Model file for the job. Use its own axes, mm. A direction names the side the tool comes from. Round coordinates to 2 decimals unless told otherwise and drop trailing zeros. Write each loop counter-clockwise with the first axis right and the second up, starting at its lowest first coordinate (ties: lowest second). Pieces come first, ordered by that corner, then holes. Notation, with made-up numbers: (-19, -35) - (23, -35) arc R21 ccw to (23, -20) - close; hole circle Ø9 at (67, -16.75). An arc over 180 degrees is marked (long way). One line per item, written item: value.
from build123d import *

# Parameters (mm, degrees)
F0_R      = 45
F1_DEPTH  = 10
F2_R      = 24.5
F2_R_2    = 20
F3_DEPTH  = 140
F4_R      = 45
F4_R_2    = 24.5
F4_R_3    = 20
F5_DEPTH  = 10
F8_DEPTH  = 195
F10_DEPTH = 18.5
F11_R     = 18.499
F12_R     = 28.5
F13_DEPTH = 10
F15_DEPTH = 25
F16_R     = 14
F17_DEPTH = 99.7
F18_R     = 20
F19_DEPTH = 202.6


# Not quite as in the source:
# - a fillet or chamfer is up to 0.001 mm smaller than in the source, because OpenCascade refuses the exact size


with BuildPart() as f1:
    # F0 (on Top) → F1 (new body)
    with BuildSketch(Plane.XY):
        Circle(F0_R)
    extrude(amount=F1_DEPTH)

    # F2 (on face) → F3 (join)
    with BuildSketch(Plane.XY.offset(10)):
        Circle(F2_R)
        Circle(F2_R_2, mode=Mode.SUBTRACT)
        Circle(F2_R_2)
    extrude(amount=F3_DEPTH)

    # F4 (on face) → F5 (join)
    with BuildSketch(Plane.XY.offset(150)):
        Circle(F4_R)
        Circle(F4_R_2, mode=Mode.SUBTRACT)
        Circle(F4_R_2)
        Circle(F4_R_3, mode=Mode.SUBTRACT)
        Circle(F4_R_3)
    extrude(amount=F5_DEPTH)

    # F7 (on face) → F8 (cut)
    with BuildSketch(Plane(origin=(0, 0, 0), x_dir=(1, 0, 0), z_dir=(0, 0, -1))):
        with BuildLine():
            ThreePointArc((-34.7419642857, -4.2421595409), (-35, 0), (-34.7419642857, 4.2421595409))
            ThreePointArc((-34.7419642857, 4.2421595409), (-39.25, 0), (-34.7419642857, -4.2421595409))
        make_face()
        with BuildLine():
            ThreePointArc((-30.75, 0), (-31.904911004, 2.9125459837), (-34.7419642857, 4.2421595409))
            ThreePointArc((-34.7419642857, 4.2421595409), (-35, 0), (-34.7419642857, -4.2421595409))
            ThreePointArc((-34.7419642857, -4.2421595409), (-31.904911004, -2.9125459837), (-30.75, 0))
        make_face()
        with BuildLine():
            ThreePointArc((-4.2421595409, -34.7419642857), (0, -35), (4.2421595409, -34.7419642857))
            ThreePointArc((4.2421595409, -34.7419642857), (0, -30.75), (-4.2421595409, -34.7419642857))
        make_face()
        with BuildLine():
            ThreePointArc((4.25, -35), (4.248039433, -34.8709225982), (4.2421595409, -34.7419642857))
            ThreePointArc((4.2421595409, -34.7419642857), (0, -35), (-4.2421595409, -34.7419642857))
            ThreePointArc((-4.2421595409, -34.7419642857), (-0.1290774018, -39.248039433), (4.25, -35))
        make_face()
        with BuildLine():
            ThreePointArc((34.7419642857, -4.2421595409), (34.935431513, -2.125), (35, 0))
            ThreePointArc((35, 0), (34.935431513, 2.125), (34.7419642857, 4.2421595409))
            ThreePointArc((34.7419642857, 4.2421595409), (30.75, 0), (34.7419642857, -4.2421595409))
        make_face()
        with BuildLine():
            ThreePointArc((34.7419642857, 4.2421595409), (34.935431513, 2.125), (35, 0))
            ThreePointArc((35, 0), (34.935431513, -2.125), (34.7419642857, -4.2421595409))
            ThreePointArc((34.7419642857, -4.2421595409), (37.9125459837, -3.095088996), (39.25, 0))
            ThreePointArc((39.25, 0), (37.9125459837, 3.095088996), (34.7419642857, 4.2421595409))
        make_face()
        with BuildLine():
            ThreePointArc((24.7487373415, 24.7487373415), (26.2056824365, 23.2004786165), (27.5659383164, 21.5666187599))
            ThreePointArc((27.5659383164, 21.5666187599), (28.6240182438, 23.0038310608), (28.9987373415, 24.7487373415))
            ThreePointArc((28.9987373415, 24.7487373415), (26.2551396829, 28.7228098102), (21.5666187599, 27.5659383164))
            ThreePointArc((21.5666187599, 27.5659383164), (23.2004786165, 26.2056824365), (24.7487373415, 24.7487373415))
        make_face()
        with BuildLine():
            ThreePointArc((21.7435335215, 21.7435335215), (24.6196599397, 20.5006979085), (27.5659383164, 21.5666187599))
            ThreePointArc((27.5659383164, 21.5666187599), (26.2056824365, 23.2004786165), (24.7487373415, 24.7487373415))
            Line((24.7487373415, 24.7487373415), (21.7435335215, 21.7435335215))
        make_face()
        with BuildLine():
            Line((21.7435335215, 21.7435335215), (24.7487373415, 24.7487373415))
            ThreePointArc((24.7487373415, 24.7487373415), (23.2004786165, 26.2056824365), (21.5666187599, 27.5659383164))
            ThreePointArc((21.5666187599, 27.5659383164), (20.5006979085, 24.6196599397), (21.7435335215, 21.7435335215))
        make_face()
        with BuildLine():
            ThreePointArc((28.9987373415, -24.7487373415), (28.6240182438, -23.0038310608), (27.5659383164, -21.5666187599))
            ThreePointArc((27.5659383164, -21.5666187599), (26.2056824365, -23.2004786165), (24.7487373415, -24.7487373415))
            ThreePointArc((24.7487373415, -24.7487373415), (23.2004786165, -26.2056824365), (21.5666187599, -27.5659383164))
            ThreePointArc((21.5666187599, -27.5659383164), (26.2551396829, -28.7228098102), (28.9987373415, -24.7487373415))
        make_face()
        with BuildLine():
            ThreePointArc((21.5666187599, -27.5659383164), (23.2004786165, -26.2056824365), (24.7487373415, -24.7487373415))
            Line((24.7487373415, -24.7487373415), (21.7435335215, -21.7435335215))
            ThreePointArc((21.7435335215, -21.7435335215), (20.5006979085, -24.6196599397), (21.5666187599, -27.5659383164))
        make_face()
        with BuildLine():
            ThreePointArc((24.7487373415, -24.7487373415), (26.2056824365, -23.2004786165), (27.5659383164, -21.5666187599))
            ThreePointArc((27.5659383164, -21.5666187599), (24.6196599397, -20.5006979085), (21.7435335215, -21.7435335215))
            Line((21.7435335215, -21.7435335215), (24.7487373415, -24.7487373415))
        make_face()
        with BuildLine():
            ThreePointArc((-27.5659383164, -21.5666187599), (-27.7539411616, -27.7539411616), (-21.5666187599, -27.5659383164))
            ThreePointArc((-21.5666187599, -27.5659383164), (-23.2004786165, -26.2056824365), (-24.7487373415, -24.7487373415))
            ThreePointArc((-24.7487373415, -24.7487373415), (-26.2056824365, -23.2004786165), (-27.5659383164, -21.5666187599))
        make_face()
        with BuildLine():
            Line((-24.7487373415, -24.7487373415), (-21.7435335215, -21.7435335215))
            ThreePointArc((-21.7435335215, -21.7435335215), (-24.6196599397, -20.5006979085), (-27.5659383164, -21.5666187599))
            ThreePointArc((-27.5659383164, -21.5666187599), (-26.2056824365, -23.2004786165), (-24.7487373415, -24.7487373415))
        make_face()
        with BuildLine():
            ThreePointArc((-20.4987373415, -24.7487373415), (-20.8222493284, -23.122332754), (-21.7435335215, -21.7435335215))
            Line((-21.7435335215, -21.7435335215), (-24.7487373415, -24.7487373415))
            ThreePointArc((-24.7487373415, -24.7487373415), (-23.2004786165, -26.2056824365), (-21.5666187599, -27.5659383164))
            ThreePointArc((-21.5666187599, -27.5659383164), (-20.7746648729, -26.2551396829), (-20.4987373415, -24.7487373415))
        make_face()
        with BuildLine():
            ThreePointArc((-24.7487373415, 24.7487373415), (-23.2004786165, 26.2056824365), (-21.5666187599, 27.5659383164))
            ThreePointArc((-21.5666187599, 27.5659383164), (-27.7539411616, 27.7539411616), (-27.5659383164, 21.5666187599))
            ThreePointArc((-27.5659383164, 21.5666187599), (-26.2056824365, 23.2004786165), (-24.7487373415, 24.7487373415))
        make_face()
        with BuildLine():
            ThreePointArc((-20.4987373415, 24.7487373415), (-20.7746648729, 26.2551396829), (-21.5666187599, 27.5659383164))
            ThreePointArc((-21.5666187599, 27.5659383164), (-23.2004786165, 26.2056824365), (-24.7487373415, 24.7487373415))
            Line((-24.7487373415, 24.7487373415), (-21.7435335215, 21.7435335215))
            ThreePointArc((-21.7435335215, 21.7435335215), (-20.8222493284, 23.122332754), (-20.4987373415, 24.7487373415))
        make_face()
        with BuildLine():
            ThreePointArc((-27.5659383164, 21.5666187599), (-24.6196599397, 20.5006979085), (-21.7435335215, 21.7435335215))
            Line((-21.7435335215, 21.7435335215), (-24.7487373415, 24.7487373415))
            ThreePointArc((-24.7487373415, 24.7487373415), (-26.2056824365, 23.2004786165), (-27.5659383164, 21.5666187599))
        make_face()
        with BuildLine():
            ThreePointArc((-4.2421595409, 34.7419642857), (0, 30.75), (4.2421595409, 34.7419642857))
            ThreePointArc((4.2421595409, 34.7419642857), (0, 35), (-4.2421595409, 34.7419642857))
        make_face()
        with BuildLine():
            ThreePointArc((-4.2421595409, 34.7419642857), (0, 35), (4.2421595409, 34.7419642857))
            ThreePointArc((4.2421595409, 34.7419642857), (4.248039433, 34.8709225982), (4.25, 35))
            ThreePointArc((4.25, 35), (-0.1290774018, 39.248039433), (-4.2421595409, 34.7419642857))
        make_face()
    extrude(amount=-F8_DEPTH, mode=Mode.SUBTRACT)

    # F9 (on Front) → F10 (join, symmetric)
    with BuildSketch(Plane.XZ):
        Polygon((-76.7210857587, 90.5581348548), (0, 13.8370490961), (0, 40), (-63.6396103068, 103.6396103068), align=None)
        Polygon((0, 40), (0, 13.8370490961), (6.2413537338, 59.9215971701), (0, 66.1629509039), align=None)
        Polygon((-63.6396103068, 103.6396103068), (0, 40), (0, 66.1629509039), (-50.5581348548, 116.7210857587), align=None)
    extrude(amount=F10_DEPTH, both=True)

    # F11 (radius 18.5 in the source; OpenCascade refuses exactly that, so slightly less here)
    f11_edges = [f1.edges().sort_by_distance(p)[0] for p in [
        (-46.391732, 18.5, 60.228781),
        (-46.391732, -18.5, 60.228781),
        (-33.310257, -18.5, 99.473208),
        (-33.310257, 18.5, 99.473208),
    ]]
    fillet(f11_edges, radius=F11_R)

    # F12 (on face) → F13 (join)
    with BuildSketch(Plane(origin=(-83.6396103068, 0, 83.6396103068), x_dir=(0, -1, 0), z_dir=(-0.7071067812, 0, 0.7071067812))):
        with Locations((0, 28.2842712475)):
            Circle(F12_R)
    extrude(amount=F13_DEPTH)

    # F14 (on face) → F15 (cut)
    with BuildSketch(Plane(origin=(-90.7106781187, 0, 90.7106781187), x_dir=(0, -1, 0), z_dir=(-0.7071067812, 0, 0.7071067812))):
        with BuildLine():
            ThreePointArc((-2.24742029, 51.6765584815), (0, 49.5342712475), (2.24742029, 51.6765584815))
            ThreePointArc((2.24742029, 51.6765584815), (0, 51.7842712475), (-2.24742029, 51.6765584815))
        make_face()
        with BuildLine():
            ThreePointArc((-2.24742029, 51.6765584815), (0, 51.7842712475), (2.24742029, 51.6765584815))
            ThreePointArc((2.24742029, 51.6765584815), (2.2493549801, 51.7303994207), (2.25, 51.7842712475))
            ThreePointArc((2.25, 51.7842712475), (-0.0538718267, 54.0336262275), (-2.24742029, 51.6765584815))
        make_face()
        with BuildLine():
            ThreePointArc((-23.392287234, 26.0368509574), (-23.5, 28.2842712475), (-23.392287234, 30.5316915375))
            ThreePointArc((-23.392287234, 30.5316915375), (-25.75, 28.2842712475), (-23.392287234, 26.0368509574))
        make_face()
        with BuildLine():
            ThreePointArc((-21.25, 28.2842712475), (-21.8713727063, 29.8367122732), (-23.392287234, 30.5316915375))
            ThreePointArc((-23.392287234, 30.5316915375), (-23.5, 28.2842712475), (-23.392287234, 26.0368509574))
            ThreePointArc((-23.392287234, 26.0368509574), (-21.8713727063, 26.7318302218), (-21.25, 28.2842712475))
        make_face()
        with BuildLine():
            ThreePointArc((-2.24742029, 4.8919840134), (0, 4.7842712475), (2.24742029, 4.8919840134))
            ThreePointArc((2.24742029, 4.8919840134), (0, 7.0342712475), (-2.24742029, 4.8919840134))
        make_face()
        with BuildLine():
            ThreePointArc((2.25, 4.7842712475), (2.2493549801, 4.8381430742), (2.24742029, 4.8919840134))
            ThreePointArc((2.24742029, 4.8919840134), (0, 4.7842712475), (-2.24742029, 4.8919840134))
            ThreePointArc((-2.24742029, 4.8919840134), (-0.0538718267, 2.5349162674), (2.25, 4.7842712475))
        make_face()
        with BuildLine():
            ThreePointArc((23.392287234, 26.0368509574), (23.4730563626, 27.1592712475), (23.5, 28.2842712475))
            ThreePointArc((23.5, 28.2842712475), (23.4730563626, 29.4092712475), (23.392287234, 30.5316915375))
            ThreePointArc((23.392287234, 30.5316915375), (21.25, 28.2842712475), (23.392287234, 26.0368509574))
        make_face()
        with BuildLine():
            ThreePointArc((23.392287234, 30.5316915375), (23.4730563626, 29.4092712475), (23.5, 28.2842712475))
            ThreePointArc((23.5, 28.2842712475), (23.4730563626, 27.1592712475), (23.392287234, 26.0368509574))
            ThreePointArc((23.392287234, 26.0368509574), (25.0524410257, 26.6556439538), (25.75, 28.2842712475))
            ThreePointArc((25.75, 28.2842712475), (25.0524410257, 29.9128985411), (23.392287234, 30.5316915375))
        make_face()
    extrude(amount=-F15_DEPTH, mode=Mode.SUBTRACT)

    # F16 (on face) → F17 (cut)
    with BuildSketch(Plane(origin=(-90.7106781187, 0, 90.7106781187), x_dir=(0, -1, 0), z_dir=(-0.7071067812, 0, 0.7071067812))):
        with Locations((0, 28.2842712475)):
            Circle(F16_R)
    extrude(amount=-F17_DEPTH, mode=Mode.SUBTRACT)

    # F18 (on face) → F19 (cut)
    with BuildSketch(Plane.XY.offset(160)):
        Circle(F18_R)
    extrude(amount=-F19_DEPTH, mode=Mode.SUBTRACT)


solid = f1.part
1. Drop flat-ended pins along their axis: pin 1 (8 mm diameter, centred on x = 17.5, z = 125.5, fed in from +Y); pin 2 (7.5 mm diameter, centred on x = -35, y = 0, fed in from -Z); pin 3 (8 mm diameter, centred on y = -15, z = 71.5, fed in from +X). Give the stop position or say it passes through.
Report:
pin 1: y = 20.45
pin 2: z = 45.09
pin 3: x = 21.89
2. Band-saw the part on B-B on y = -11.5. Write the cut outline in (x, z).
Report:
outline: (-89.15, 92.27) - (-82.08, 85.2) - (-73.89, 93.39) - (-21.63, 41.14) - (-21.63, 10) - (-43.51, 10) - (-43.51, 0) - (-16.36, 0) - (-16.36, 45.07) - (-76.36, 105.06) - close; (-65.06, 116.36) - (-16.36, 67.65) - (-16.36, 160) - (-43.51, 160) - (-43.51, 150) - (-21.63, 150) - (-21.63, 82.13) - (-53.39, 113.89) - (-45.2, 122.08) - (-52.27, 129.15) - close; (16.36, 0) - (43.51, 0) - (43.51, 10) - (21.63, 10) - (21.63, 150) - (43.51, 150) - (43.51, 160) - (16.36, 160) - close
3. Mould opens along Y. For faces 6 (the face through (-74.91, 13.07, 106.51)), 7 (the face through (-38.37, 2.59, 154.93)), 8 (the face through (20.765, -39.923, 4.93)) say: released by +Y, released by -Y, zero draft, split by the parting line, or undercut.
Report:
face 6: zero draft
face 7: undercut
face 8: split by the parting line
4. Band-saw the part on C-C on z = 21. Write the cut outline in (x, y).
Report:
outline: circle Ø49 at (0, 0); hole circle Ø40 at (0, 0)
5. Wall check: probe 1 along Z at (x, y) = (14.5, 32); probe 2 along X at (y, z) = (0, 88); probe 3 along X at (y, z) = (11, 72.5). Give the ranges that are in metal, low to high. Write a range as [from, to].
Report:
probe 1: [0, 10], [150, 160]
probe 2: [-88.31, -84.42], [-74.16, -67.8], [-28.2, -20], [20, 24.5]
probe 3: [-53.54, -44.75], [-20.25, -16.7], [16.7, 21.89]
6. Tool access for faces 1 (the face through (-38.37, 2.59, 4.93)), 2 (the face through (-46.48, 12.94, 67.78)), 3 (the face through (-46.48, -12.94, 67.78)), 4 (the face through (19, -19, 10)), 5 (the face through (9, -19, 160)): list every direction of +Z, -Z, +X, -X, +Y, -Y with a clear straight run to the whole face (end or side of a thin tool).
Report:
face 1: -Z
face 2: +Y
face 3: -Y
face 4: none
face 5: +Z, +X, -X, +Y, -Y
7. Band-saw the part on A-A on x = 0. State how many separate pieces and enclosed holes the cut face has, plus the area to 3 significant figures.
Report:
separate pieces: 6
enclosed holes: 0
area: 1,920 mm²
